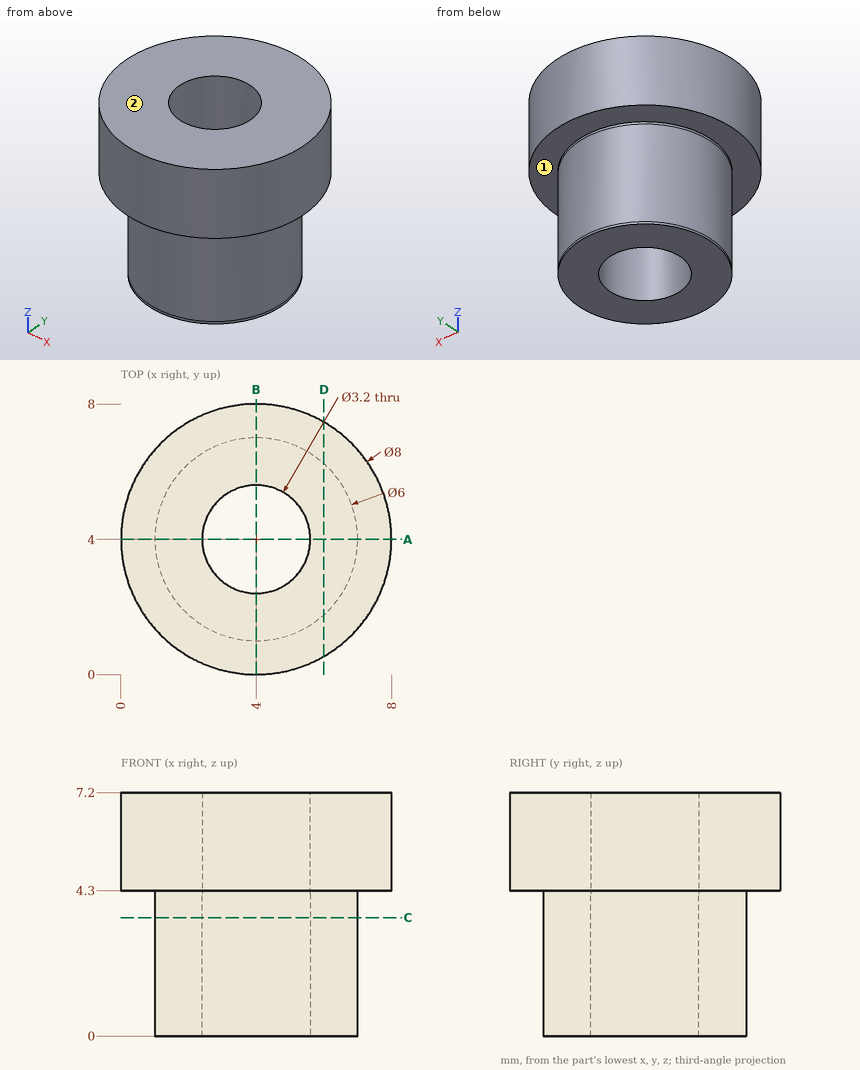
Could you check a few things on this drawing? It's one solid part, dimensions in mm from its lowest x, y, z. A direction names the side the tool comes from. Coordinates: 2 decimals unless noted, no trailing zeros. Write each loop counter-clockwise with the first axis right and the second up, starting at its lowest first coordinate (ties: lowest second). Pieces come first, ordered by that corner, then holes.
Q1. Which directions (+Z, -Z, +X, -X, +Y, -Y) give clear straight access to the entire face, cutting with the end or side of a thin tool? Please do the marked faces 1 and 2.
Results found:
face 1: -Z
face 2: +Z, +X, -X, +Y, -Y
Q2. Please list where these lines run through material, in increasing order: L1, parallel to Y at x = 4, z = 1.8; L2, parallel to Y at x = 4, z = 6.2; L3, parallel to X at y = 4.75, z = 0.5.
Results found:
L1: y = 1 to 2.4, 5.6 to 7
L2: y = 0 to 2.4, 5.6 to 8
L3: x = 1.1 to 2.59, 5.41 to 6.9
Q3. Imagine slicing it at A-A, the plane y = 4. List the corners of the cut face in (x, z) for me, plus the area to 3 significant figures.
Results found:
outline: (0, 4.3) - (1, 4.3) - (1, 0) - (2.4, 0) - (2.4, 7.2) - (0, 7.2) - close; (5.6, 0) - (7, 0) - (7, 4.3) - (8, 4.3) - (8, 7.2) - (5.6, 7.2) - close
area: 26.0 mm2
Q4. Imagine slicing it at C-C, the plane z = 3.5. List the corners of the cut face in (x, y) for me.
Results found:
outline: circle Ø6 at (4, 4); hole circle Ø3.2 at (4, 4)
Q5. For P1, Ø1.5, axis at y = 3.5, z = 1.5, coming from the +X side; P2, Ø2.5, axis at x = 4, y = 4, coming from the +Z side, each with a flat end and sliding along its axis, tell me the tip position at first contact or that it passes through.
Results found:
P1: stops at x = 7
P2: passes through
Q6. Imagine slicing it at D-D, the plane x = 6. List the corners of the cut face in (y, z) for me.
Results found:
outline: (0.54, 4.3) - (1.76, 4.3) - (1.76, 0) - (6.24, 0) - (6.24, 4.3) - (7.46, 4.3) - (7.46, 7.2) - (0.54, 7.2) - close
